Work out the finished part from the listing and answer in its coordinate system (mm). A direction names the side the tool comes from. Round coordinates to 2 decimals unless told otherwise and drop trailing zeros. Loops run counter-clockwise (first coordinate to the right, second up) from the corner with the lowest first, then second, coordinate; pieces in that order, holes last. Notation, with made-up numbers: (-29.75, 65) - (-25.75, 65) arc R11 ccw to (-25.75, 70) - close; hole circle Ø2 at (40, -1). An arc over 180 degrees is marked (long way). Answer as CSV lines item,"result". Start each with the question number.
Q1. Straight lines are drawn through the part: L1, parallel to X at y = 14.5, z = -8.5; L2, parallel to Y at x = 2, z = -5.5; L3, parallel to X at y = 21.5, z = -5.25. For each, find the intervals that lie inside material, in ascending order. Write a range as [from, to].
Q2. The mould has two halves that part along X. Classify faces 1 (the face through (-4, 13, -6)), 2 (the face through (31, 25, -6)), 3 (the face through (28, 15, -6)): +X half, -X half, draft (parallel to the pull), parting line (faces both ways), or undercut.
Q3. Section A-A on y = 21 is taken. Write down the section's boundary in (x, z).
Q4. For faces 4 (the face through (16, 0, -6)), 5 (the face through (31, 10, -6)), 6 (the face through (1, 25, -6)), 7 (the face through (16, 4, 2.5)), 8 (the face through (26, 20, -6)), determine the directions among +Z, -Z, +X, -X, +Y, -Y from which every point of the face is accessible in a straight line to the end or side of a thin tool.
Q5. Section C-C on y = -7 is taken. Write down the section's boundary in (x, z).
Q6. Section B-B on z = -6 is taken. Write down the section's boundary in (x, y), then the cut area to 3 significant figures.
Q7. Each of these flat-tipped pins is pushed along its axis until it touches: pin 1 Ø1.5 at (x, z) = (28, -3) entering from -Y; pin 2 Ø10 at (x, z) = (16, -11) entering from -Y; pin 3 Ø5 at (x, z) = (21.5, -2.5) entering from +Y. Where does it stop, or does it pass through?
```python
from build123d import *
from build123d.topology import SkipClean

# Parameters (mm, degrees)
SKETCH_3_W          = 32
SKETCH_3_H          = 12
EXTRUDE_3_DEPTH     = 5
SKETCH_4_R          = 5
EXTRUDE_4_DEPTH     = 10
SKETCH_8_R          = 5
EXTRUDE_6_DEPTH     = 5
SKETCH_9_R          = 4.8
CUT_EXTRUDE_2_DEPTH = 0.5
EXTRUDE_START       = 5
SKETCH_36_R         = 5
SKETCH_36_R_2       = 4.98
EXTRUDE_11_DEPTH    = 5
SKETCH_46_W         = 32
SKETCH_46_H         = 12
EXTRUDE_12_DEPTH    = 20
SKETCH_47_W         = 4
SKETCH_47_H         = 25
EXTRUDE_13_DEPTH    = 12
SKETCH_48_W         = 4
SKETCH_48_H         = 25
EXTRUDE_14_DEPTH    = 12
CUT_EXTRUDE_START   = -12
CUT_EXTRUDE_5_DEPTH = 12
SKETCH_50_R         = 6
EXTRUDE_15_DEPTH    = 20
SKETCH_51_R         = 6
EXTRUDE_16_DEPTH    = 20
EXTRUDE_17_DEPTH    = 2.5
EXTRUDE_18_DEPTH    = 2.5


# Read off the part's stored shape, not the designer's step: the extrude step
with BuildPart() as part:
    # Sketch 3 → Extrude 3 (new body)
    with BuildSketch(Plane(origin=(0, 0, 0), x_dir=(1, 0, 0), z_dir=(0, 1, 0))):
        with Locations((16, 6)):
            Rectangle(SKETCH_3_W, SKETCH_3_H)
    extrude(amount=EXTRUDE_3_DEPTH)

    # Sketch 4 → Extrude 4 (add)
    with BuildSketch(Plane.XZ):
        with Locations(Location((6, -6, 0), (0, 0, 270))):
            Circle(SKETCH_4_R)
        with Locations(Location((26, -6, 0), (0, 0, 270))):
            Circle(SKETCH_4_R)
    extrude(amount=EXTRUDE_4_DEPTH)

    # Sketch 8 → Extrude 6 (add)
    with BuildSketch(Plane.XZ.offset(10)):
        with Locations(Location((6, -6, 0), (0, 0, 270))):
            Circle(SKETCH_8_R)
    extrude(amount=EXTRUDE_6_DEPTH)

    # Sketch 9 → Cut-Extrude 2 (cut)
    with BuildSketch(Plane.XZ.offset(15)):
        with Locations(Location((6, -6, 0), (0, 0, 270))):
            Circle(SKETCH_9_R)
    extrude(amount=-CUT_EXTRUDE_2_DEPTH, mode=Mode.SUBTRACT)



with BuildPart() as body_2:
    # Sketch 14 → Revolve 2 (revolve)
    with BuildSketch(Plane.XY.offset(-6), mode=Mode.PRIVATE) as revolve_2_sk:
        Polygon((1.021282046, -15), (1.021282046, -20), (1.221282046, -15), align=None)
    revolve(revolve_2_sk.sketch.rotate(Axis((6, -15, -6), (0, 1, 0)), 270), axis=Axis((6, -15, -6), (0, 1, 0)))


with BuildPart() as part_1:
    with SkipClean():  # the faces are left unmerged after this step: merging them gives an invalid solid
        add(part.part)

        add(body_2.part)  # Extrude 11 merges body 2
        # Sketch 36 → Extrude 11 (add)
        with BuildSketch(Plane(origin=(0, -20, 0), x_dir=(1, 0, 0), z_dir=(0, 1, 0)).offset(EXTRUDE_START)):
            with Locations(Location((6, 6, 0), (0, 0, 270))):
                Circle(SKETCH_36_R)
            with Locations(Location((6, 6, 0), (0, 0, 90))):
                Circle(SKETCH_36_R_2, mode=Mode.SUBTRACT)
        extrude(amount=-EXTRUDE_11_DEPTH)

    # Sketch 46 → Extrude 12 (add)
    with SkipClean():  # the faces are left unmerged after this step: merging them gives an invalid solid
        with BuildSketch(Plane(origin=(0, 5, 0), x_dir=(1, 0, 0), z_dir=(0, 1, 0))):
            with Locations((16, 6)):
                Rectangle(SKETCH_46_W, SKETCH_46_H)
        extrude(amount=EXTRUDE_12_DEPTH)

    # Sketch 47 → Extrude 13 (add)
    with SkipClean():  # the faces are left unmerged after this step: merging them gives an invalid solid
        with BuildSketch(Plane.XY):
            with Locations((-2, 12.5)):
                Rectangle(SKETCH_47_W, SKETCH_47_H)
        extrude(amount=-EXTRUDE_13_DEPTH)

    # Sketch 48 → Extrude 14 (add)
    with SkipClean():  # the faces are left unmerged after this step: merging them gives an invalid solid
        with BuildSketch(Plane.XY):
            with Locations((34, 12.5)):
                Rectangle(SKETCH_48_W, SKETCH_48_H)
        extrude(amount=-EXTRUDE_14_DEPTH)

    # Cut-Extrude 5 outline → Cut-Extrude 5 (cut)
    with SkipClean():  # the faces are left unmerged after this step: merging them gives an invalid solid
        with BuildSketch(Plane.XY.offset(CUT_EXTRUDE_START)):
            Polygon((26, 25), (6, 25), (6, 15), (1, 15), (1, 5), (31, 5), (31, 15), (26, 15), align=None)
        extrude(amount=CUT_EXTRUDE_5_DEPTH, mode=Mode.SUBTRACT)

    # Sketch 50 → Extrude 15 (add)
    with BuildSketch(Plane.XZ):
        with Locations(Location((6, -6, 0), (0, 0, 270))):
            Circle(SKETCH_50_R)
    extrude(amount=EXTRUDE_15_DEPTH)

    # Sketch 51 → Extrude 16 (add)
    with BuildSketch(Plane.XZ):
        with Locations(Location((26, -6, 0), (0, 0, 270))):
            Circle(SKETCH_51_R)
    extrude(amount=EXTRUDE_16_DEPTH)

    # Sketch 52 → Revolve 3 (revolve)
    with BuildSketch(Plane.XY.offset(-6), mode=Mode.PRIVATE) as revolve_3_sk:
        Polygon((0, -20), (0, -25), (0.2, -20), align=None)
    revolve(revolve_3_sk.sketch.rotate(Axis((6, -20, -6), (0, -1, 0)), 270), axis=Axis((6, -20, -6), (0, -1, 0)))

    # Sketch 53 → Revolve 4 (revolve)
    with BuildSketch(Plane.XY.offset(-6), mode=Mode.PRIVATE) as revolve_4_sk:
        Polygon((20, -20), (20, -25), (20.2, -20), align=None)
    revolve(revolve_4_sk.sketch.rotate(Axis((26, -20, -6), (0, -1, 0)), 270), axis=Axis((26, -20, -6), (0, -1, 0)))

    # Sketch 55 → Extrude 17 (add)
    with BuildSketch(Plane.XY):
        Polygon((-4, 25), (6, 25), (6, 15), (1, 15), (1, 5), (31, 5), (31, 15), (26, 15), (26, 25), (36, 25), (36, 0), (-4, 0), align=None)
    extrude(amount=EXTRUDE_17_DEPTH)

    # Sketch 56 → Extrude 18 (add)
    with BuildSketch(Plane(origin=(0, 0, -12), x_dir=(-1, 0, 0), z_dir=(0, 0, -1))):
        Polygon((-36, 25), (-26, 25), (-26, 15), (-31, 15), (-31, 5), (-1, 5), (-1, 15), (-6, 15), (-6, 25), (4, 25), (4, 0), (-36, 0), align=None)
    extrude(amount=EXTRUDE_18_DEPTH)


solid = part_1.part
```
Findings:
1,L1,"x = [-4, 1], [31, 36]"
1,L2,"y = [-20, 5], [15, 25]"
1,L3,"x = [-4, 6], [26, 36]"
2,face 1,"-X half"
2,face 2,"draft"
2,face 3,"undercut"
3,outline,"(-4, -14.5) - (6, -14.5) - (6, 2.5) - (-4, 2.5) - close; (26, -14.5) - (36, -14.5) - (36, 2.5) - (26, 2.5) - close"
4,face 4,"-Y"
4,face 5,"+Z, -Z"
4,face 6,"+Z, -Z, +X, -X, +Y"
4,face 7,"+Z, +X, -X, +Y, -Y"
4,face 8,"+Z, -Z, +Y"
5,outline,"circle Ø12 at (6, -6); circle Ø12 at (26, -6)"
6,outline,"(-4, 0) - (0, 0) - (0, -25) - (0.2, -20) - (11.8, -20) - (12, -25) - (12, 0) - (20, 0) - (20, -25) - (20.2, -20) - (31.8, -20) - (32, -25) - (32, 0) - (36, 0) - (36, 25) - (26, 25) - (26, 15) - (31, 15) - (31, 5) - (1, 5) - (1, 15) - (6, 15) - (6, 25) - (-4, 25) - close"
6,area,"982 mm^2"
7,pin 1,"stops at y = -20"
7,pin 2,"stops at y = 0"
7,pin 3,"stops at y = 5"
